```python
from build123d import *

# Parameters (mm, degrees)
ESQUISSE1_W             = 18
ESQUISSE1_H             = 18
BOSS_EXTRU_1_DEPTH      = 20
ENL_V_MAT_EXTRU_1_DEPTH = 20
ENL_V_START             = -2
ENL_V_MAT_EXTRU_2_DEPTH = 16
CHANFREIN1_SIZE         = 0.5
ESQUISSE4_R             = 2
ENL_V_MAT_EXTRU_3_DEPTH = 4
ESQUISSE5_R             = 2
ENL_V_MAT_EXTRU_4_DEPTH = 4


with BuildPart() as part:
    # Esquisse1 → Boss.-Extru.1 (new body)
    with BuildSketch(Plane.XY):
        with Locations((9, 9)):
            Rectangle(ESQUISSE1_W, ESQUISSE1_H)
    extrude(amount=BOSS_EXTRU_1_DEPTH)

    # Esquisse2 → Enlèv. mat.-Extru.1 (cut)
    with BuildSketch(Plane.XY.offset(20)):
        Polygon((18, 18), (2, 18), (18, 2), align=None)
    extrude(amount=-ENL_V_MAT_EXTRU_1_DEPTH, mode=Mode.SUBTRACT)

    # Esquisse3 → Enlèv. mat.-Extru.2 (cut)
    with BuildSketch(Plane.XY.offset(20).offset(ENL_V_START)):
        Polygon((3, 17), (3, 3), (17, 3), align=None)
    extrude(amount=-ENL_V_MAT_EXTRU_2_DEPTH, mode=Mode.SUBTRACT)

    # Chanfrein1
    chanfrein1_edges = [part.edges().sort_by_distance(p)[0] for p in [
        (0, 18, 10),
        (18, 0, 10),
        (0, 0, 10),
    ]]
    chamfer(chanfrein1_edges, length=CHANFREIN1_SIZE)

    # Esquisse4 → Enlèv. mat.-Extru.3 (cut, through all)
    with BuildSketch(Plane(origin=(3, 0, 0), x_dir=(0, 0, -1), z_dir=(1, 0, 0))):
        with Locations((-10, 11)):
            Circle(ESQUISSE4_R)
    extrude(amount=-ENL_V_MAT_EXTRU_3_DEPTH, mode=Mode.SUBTRACT)

    # Esquisse5 → Enlèv. mat.-Extru.4 (cut, through all)
    with BuildSketch(Plane(origin=(0, 3, 0), x_dir=(1, 0, 0), z_dir=(0, 1, 0))):
        with Locations((11, -10)):
            Circle(ESQUISSE5_R)
    extrude(amount=-ENL_V_MAT_EXTRU_4_DEPTH, mode=Mode.SUBTRACT)


solid = part.part
```
For this review, take the finished solid that the model builds, in its own axes (mm). A direction names the side the tool comes from. Round coordinates to 2 decimals unless told otherwise and drop trailing zeros. Write each loop counter-clockwise with the first axis right and the second up, starting at its lowest first coordinate (ties: lowest second). Pieces come first, ordered by that corner, then holes. Notation, with made-up numbers: (-36, 67) -> (-29, 67) arc R5 cw to (-29, 73) -> close; hole circle Ø7 at (72.5, -2.5). An arc over 180 degrees is marked (long way). One line per question, with ' | ' between items. Start each with the question number.
(1) Tool access review of faces 1 (the face through (18, 1, 10)), 2 (the face through (7, 7, 18)): name each direction out of +Z, -Z, +X, -X, +Y, -Y from which nothing blocks a thin tool from reaching the whole face with its end or side.
(2) For line 1 along Z through (x, y) = (8.25, 7); line 2 along Y through (x, z) = (0.85, 10); line 3 along Z through (x, y) = (11, 2.1), list the stretches that pass through material, from the lowest coordinate up. Write a range as from..to.
(3) Insertion check: P1, Ø5, axis at x = 5, z = 17, coming from the +Y side; P2, Ø4, axis at x = 11.5, z = 11.5, coming from the +Y side; P3, Ø2.5, axis at y = 11, z = 10, coming from the +X side; P4, Ø1, axis at y = 14, z = 9.5, coming from the +X side. Each pin has a flat end and moves straight along its axis. Give the tip position at first contact, or say it passes through.
(4) Add section D-D, the plane y = 15.75. Write out the cut boundary in (x, z).
(5) Add section C-C, the plane z = 10. Write out the cut boundary in (x, y), plus the area to 3 significant figures.
(6) Mouldability with a two-part tool opening along Z and no side actions: class faces 3 (the face through (7, 7, 0)), 4 (the face through (2, 13, 10)), 5 (the face through (7, 7, 20)), 6 (the face through (10, 10, 18.2)) as released by +Z, released by -Z, zero draft, split by the parting line, or undercut.
(7) Add section A-A, the plane y = 11. Write out the cut boundary in (x, z), plus the area to 3 significant figures.
Answer list:
1) face 1: +Z, -Z, +X, +Y, -Y | face 2: +X, +Y
2) line 1: 0..2, 18..20 | line 2: 0..9, 13..18 | line 3: 0..8, 12..20
3) P1: y = 17.5 | P2: y = 3 | P3: through | P4: x = 3
4) outline: (0, 0) -> (4.25, 0) -> (4.25, 2) -> (3, 2) -> (3, 18) -> (4.25, 18) -> (4.25, 20) -> (0, 20) -> close
5) outline: (0, 0.5) -> (0.5, 0) -> (9, 0) -> (9, 3) -> (3, 3) -> (3, 9) -> (0, 9) -> close; (0, 13) -> (3, 13) -> (3, 17) -> (2, 18) -> (0.5, 18) -> (0, 17.5) -> close; (13, 0) -> (17.5, 0) -> (18, 0.5) -> (18, 2) -> (17, 3) -> (13, 3) -> close | area: 73.6 mm²
6) face 3: released by -Z | face 4: undercut | face 5: released by +Z | face 6: zero draft
7) outline: (0, 0) -> (9, 0) -> (9, 2) -> (3, 2) -> (3, 8) -> (0, 8) -> close; (0, 12) -> (3, 12) -> (3, 18) -> (9, 18) -> (9, 20) -> (0, 20) -> close | area: 72.0 mm²
